Autodesk Inventor part; units mm, degrees
ref_plane "YZ Plane" through (0, 0, 0) normal (1, 0, 0) x (0, 1, 0)
ref_plane "XZ Plane" through (0, 0, 0) normal (0, 1, 0) x (-1, 0, 0)
ref_plane "XY Plane" through (0, 0, 0) normal (0, 0, 1) x (1, 0, 0)
sketch "Boceto1" plane through (0, 0, 0) normal (0, 0, 1) x (1, 0, 0)
  circle A0 centre (0, 0) radius 6
  line L0 (-10, -32.5) -> (10, -32.5)
  line L1 (10, -32.5) -> (10, 32.5)
  line L2 (10, 32.5) -> (-10, 32.5)
  line L3 (-10, 32.5) -> (-10, -32.5)
  line L4 (-10, -32.5) -> (10, 32.5) construction
  line L5 (10, -32.5) -> (-10, 32.5) construction
  line L6 (0, 0) -> (84.0619, 0)
  line L7 (0, 0) -> (120, 0)
  circle A1 centre (120, 0) radius 6
  line L8 (110, -32.5) -> (130, -32.5)
  line L9 (130, -32.5) -> (130, 32.5)
  line L10 (130, 32.5) -> (110, 32.5)
  line L11 (110, 32.5) -> (110, -32.5)
  line L12 (110, -32.5) -> (130, 32.5) construction
  line L13 (130, -32.5) -> (110, 32.5) construction
  line L14 (10, -32.5) -> (110, -32.5)
  line L15 (110, -32.5) -> (110, -22.5)
  line L16 (110, -22.5) -> (10, -22.5)
  line L17 (110, 32.5) -> (110, 22.5)
  line L18 (110, 22.5) -> (10, 22.5)
  line L19 (10, 32.5) -> (110, 32.5)
  dimension "d0" = 12
  dimension "d1" = 120
  dimension "d2" = 65
  dimension "d3" = 20
  dimension "d4" = 20
  dimension "d5" = 65
  dimension "d6" = 10
  dimension "d7" = 10
extrude "Extrusión1" add sketch "Boceto1" along normal blind 10 contours L1 L0 L3 L2 | L16 L11 L14 L1 | L1 L19 L11 L18 | A1 | L11 L10 L9 L8
sketch "Boceto2" plane through (0, 0, 10) normal (0, 0, 1) x (1, 0, 0)
  circle A0 centre (0, 0) radius 6
  line L0 (0, 0) -> (120, 0)
  circle A1 centre (120, 0) radius 6
  dimension "d10" = 120
  dimension "d11" = 12
extrude "Extrusión2" add sketch "Boceto2" along normal blind 10 contours A1
properties part number "Eslabon_1_inventor"
Here's how the part is built. I have some questions about the finished solid (model axes, mm). A direction names the side the tool comes from. Coordinates: 2 decimals unless noted, no trailing zeros. Write each loop counter-clockwise with the first axis right and the second up, starting at its lowest first coordinate (ties: lowest second). Pieces come first, ordered by that corner, then holes. Notation, with made-up numbers: M 35.5,-29.5 L 49.5,-29.5 A15 ccw 49.5,-23.5 Z; hole C -40,-1 d4. An arc over 180 degrees is marked long. Answer as CSV lines item,"result". Start each with the question number.
Q1. Suppose I cut it at D-D, the plane y = 2.5. List the corners of the cut face in (x, z) for me, then the cut area to 3 significant figures.
Q2. If we mould it in two halves opening along Y, with no side actions, what happens to faces 1 (the flat face through (130, 0, 5)), 2 (the cylindrical face through (114, 0, 15)), 3 (the cylindrical face through (-6, 0, 5))? For each: pulls with the +Y half, pulls with the -Y half, needs draft (parallel to the pull), parting line crosses it, or undercut.
Q3. I need wall thicknesses on probe 1 along X at (y, z) = (-0.5, 5.75); probe 2 along Y at (x, z) = (0, 2.5); probe 3 along X at (y, z) = (-19, 9). Which ranges of each line are inside material? Lowest first, please. Write a range as [from, to].
Q4. Suppose I cut it at A-A, the plane x = 0. List the corners of the cut face in (y, z) for me, then the cut area to 3 significant figures.
Q5. For faces 4 (the flat face through (-10, 0, 5)), 5 (the flat face through (61, -22.5, 5)), which set-ups out of +Z, -Z, +X, -X, +Y, -Y let a thin tool reach every point of the face, with its end or its side?
Q6. Suppose I cut it at B-B, the plane y = -14. List the corners of the cut face in (x, z) for me, then the cut area to 3 significant figures.
Q7. Will these pins go through, and if not, where does the flat tip stop? pin 1 Ø7 at (x, y) = (0, 0) entering from -Z; pin 2 Ø4 at (x, z) = (113.5, 17.5) entering from -Y.
Q8. Suppose I cut it at C-C, the plane z = 1.75. List the corners of the cut face in (x, y) for me, then the cut area to 3 significant figures.
Entries:
1,outline,"M -10,0 L -5.45,0 L -5.45,10 L -10,10 Z; M 5.45,0 L 10,0 L 10,10 L 5.45,10 Z; M 110,0 L 130,0 L 130,10 L 125.45,10 L 125.45,20 L 114.55,20 L 114.55,10 L 110,10 Z"
1,area,"400 mm²"
2,face 1,"needs draft"
2,face 2,"parting line crosses it"
2,face 3,"undercut"
3,probe 1,"x = [-10, -5.98], [5.98, 10], [110, 130]"
3,probe 2,"y = [-32.5, -6], [6, 32.5]"
3,probe 3,"x = [-10, 10], [110, 130]"
4,outline,"M -32.5,0 L -6,0 L -6,10 L -32.5,10 Z; M 6,0 L 32.5,0 L 32.5,10 L 6,10 Z"
4,area,"530 mm²"
5,face 4,"+Z, -Z, -X, +Y, -Y"
5,face 5,"+Z, -Z"
6,outline,"M -10,0 L 10,0 L 10,10 L -10,10 Z; M 110,0 L 130,0 L 130,10 L 110,10 Z"
6,area,"400 mm²"
7,pin 1,"passes through"
7,pin 2,"stops at y = -3.97"
8,outline,"M -10,-32.5 L 130,-32.5 L 130,32.5 L -10,32.5 Z; hole C 0,0 d12; hole M 10,-22.5 L 110,-22.5 L 110,22.5 L 10,22.5 Z"
8,area,"4,490 mm²"
